from build123d import *

# Parameters (mm, degrees)
SKETCH4_R                  = 3
MOTOR_COOLING_SYSTEM_DEPTH = 6
SKETCH6_R                  = 3
MOTOR_BASE_HOLDER_DEPTH    = 1
SKETCH9_R                  = 1.25
SKETCH9_R_2                = 1.5
SCREWS_CUT_DEPTH           = 2


with BuildPart() as part:
    # Sketch1 → Electric motor body (revolve)
    with BuildSketch(Plane.XY):
        Polygon((0, 0), (1.585, 0), (1.585, 1), (12.5, 1), (15, 5.5), (1.585, 5.5), (1.585, 6), (15, 6), (15, 23), (10, 26.5), (5, 26.5), (5, 28.5), (1.585, 28.5), (1.585, 40.5), (0, 40.5), align=None)
    revolve(axis=Axis((0, 0, 0), (0, 1, 0)))

    # Sketch4 → motor cooling system (cut)
    with BuildSketch(Plane(origin=(0, 26.5, 0), x_dir=(1, 0, 0), z_dir=(0, 1, 0))):
        with Locations((0, -10)):
            Circle(SKETCH4_R)
        with Locations((-10, 0)):
            Circle(SKETCH4_R)
        with Locations((10, 0)):
            Circle(SKETCH4_R)
        with Locations((0, 10)):
            Circle(SKETCH4_R)
    extrude(amount=-MOTOR_COOLING_SYSTEM_DEPTH, mode=Mode.SUBTRACT)

    # Sketch6 → Motor base holder (add)
    with BuildSketch(Plane.XZ.offset(-1)):
        with BuildLine():
            Line((19.994606566, -0.5), (19.994606566, 0.5))
            ThreePointArc((19.994606566, 0.5), (19.408820128, 1.914213562), (17.994606566, 2.5))
            Line((17.994606566, 2.5), (9.994606566, 2.5))
            ThreePointArc((9.994606566, 2.5), (4.691305707, 4.696699141), (2.494606566, 10))
            Line((2.494606566, 10), (2.494606566, 18))
            ThreePointArc((2.494606566, 18), (1.908820128, 19.414213562), (0.494606566, 20))
            Line((0.494606566, 20), (-0.494606566, 20))
            ThreePointArc((-0.494606566, 20), (-1.912618477, 19.410404985), (-2.494577633, 17.989242221))
            Line((-2.494577633, 17.989242221), (-2.451820757, 10.040341672))
            ThreePointArc((-2.451820757, 10.040341672), (-4.634167594, 4.710981307), (-9.951712259, 2.5))
            Line((-9.951712259, 2.5), (-18.005393434, 2.5))
            ThreePointArc((-18.005393434, 2.5), (-19.419606996, 1.914213562), (-20.005393434, 0.5))
            Line((-20.005393434, 0.5), (-20.005393434, -0.5))
            ThreePointArc((-20.005393434, -0.5), (-19.419606996, -1.914213562), (-18.005393434, -2.5))
            Line((-18.005393434, -2.5), (-9.994606566, -2.5))
            ThreePointArc((-9.994606566, -2.5), (-4.691305707, -4.696699141), (-2.494606566, -10))
            Line((-2.494606566, -10), (-2.494606566, -18))
            ThreePointArc((-2.494606566, -18), (-1.908820128, -19.414213562), (-0.494606566, -20))
            Line((-0.494606566, -20), (0.494606566, -20))
            ThreePointArc((0.494606566, -20), (1.908820128, -19.414213562), (2.494606566, -18))
            Line((2.494606566, -18), (2.494606566, -10))
            ThreePointArc((2.494606566, -10), (4.691305707, -4.696699141), (9.994606566, -2.5))
            Line((9.994606566, -2.5), (17.994606566, -2.5))
            ThreePointArc((17.994606566, -2.5), (19.408820128, -1.914213562), (19.994606566, -0.5))
        make_face()
        Circle(SKETCH6_R, mode=Mode.SUBTRACT)
    extrude(amount=MOTOR_BASE_HOLDER_DEPTH)

    # Sketch9 → Screws cut (cut)
    with BuildSketch(Plane.XZ):
        with Locations((-17.505393434, 0)):
            Circle(SKETCH9_R)
        with Locations((17.494606566, 0)):
            Circle(SKETCH9_R)
        with Locations((0, -17.5)):
            Circle(SKETCH9_R)
        with Locations((0, 17.5)):
            Circle(SKETCH9_R)
        with Locations((7, 0)):
            Circle(SKETCH9_R_2)
        with Locations((0, -7)):
            Circle(SKETCH9_R_2)
        with Locations((-7, 0)):
            Circle(SKETCH9_R_2)
        with Locations((0, 7)):
            Circle(SKETCH9_R_2)
    extrude(amount=-SCREWS_CUT_DEPTH, mode=Mode.SUBTRACT)


solid = part.part
Input: part model. Units: mm. Frame: model coordinates. A direction names the side the tool comes from. Give positions to 0.01 mm unless a question says otherwise; leave off trailing zeros. Loops run counter-clockwise (first coordinate to the right, second up) from the corner with the lowest first, then second, coordinate; pieces in that order, holes last. Notation, with made-up numbers: (5, 80) - (39, 80) arc R29 cw to (39, 119) - close; hole circle Ø1 at (2, 40). An arc over 180 degrees is marked (long way). Use CSV: the item, a comma, the result in double quotes. Start each with the question number.
Item 1: Section A-A on y = 13. Return loops of the section in (x, z).
Item 2: Mould query, pull axis Z, two halves, no side actions, for faces 1 (the cylindrical face through (-0.65, 23.54, -7.07)), 2 (the flat face through (2, 28.5, 0)), 3 (the cylindrical face through (4.75, 0.51, 4.64)). Classes: pulls with the +Z half, pulls with the -Z half, needs draft (parallel to the pull), parting line crosses it, or undercut.
Item 3: Reachability of faces 4 (the flat face through (10, 20.5, 0)), 5 (the cylindrical face through (-1.26, 5.75, 0.96)), 6 (the cylindrical face through (-1.26, 0.51, 0.96)), 7 (the cylindrical face through (-1.924, 0.507, -19.399)), 8 (the cylindrical face through (-16.35, 0.49, -0.48)) from +Z, -Z, +X, -X, +Y, -Y: full face, straight path, thin tool, end or side. Return the list, or none.
Item 4: Contact query for flat-ended pins moving along their axis: P1, Ø6, axis at y = 13.5, z = 5, coming from the -X side; P2, Ø1, axis at y = 17.5, z = -10.5, coming from the -X side; P3, Ø1.5, axis at x = 0.5, z = 7.5, coming from the -Y side. Output: stop coordinate, or through.
Item 5: Line query: line 1 (Y direction, x = 0.5, z = -6.5); line 2 (Z direction, x = 0, y = 23); line 3 (Y direction, x = -1, z = -11). Output: solid intervals per line, ascending.
Item 6: Section B-B on y = 31. Return loops of the section in (x, z) (3 decimals).
Ans:
1,outline,"circle Ø30 at (0, 0)"
2,face 1,"undercut"
2,face 2,"needs draft"
2,face 3,"pulls with the +Z half"
3,face 4,"+Y"
3,face 5,"none"
3,face 6,"-Y"
3,face 7,"-Z, -X, +Y, -Y"
3,face 8,"+Y, -Y"
4,P1,"stops at x = -14.87"
4,P2,"stops at x = -11.18"
4,P3,"stops at y = 2"
5,line 1,"y = 2 to 5.5, 6 to 26.5"
5,line 2,"z = -15 to -13, -7 to 7, 13 to 15"
5,line 3,"y = 0 to 5.5, 6 to 20.5"
6,outline,"circle Ø3.17 at (0, 0)"
